from build123d import *

# Parameters (mm, degrees)
EXTRUDE_1_DEPTH     = 12
SKETCH_2_R          = 3
CUT_EXTRUDE_1_DEPTH = 12
FILLET_1_R          = 10
SKETCH_3_R          = 10
CUT_EXTRUDE_2_DEPTH = 12


with BuildPart() as part:
    # 草图1 → 凸台-拉伸1 (new body)
    with BuildSketch(Plane(origin=(0, 0, 0), x_dir=(1, 0, 0), z_dir=(0, 1, 0))):
        with BuildLine():
            Line((-28.145825623, 33.75), (0, 50))
            Line((0, 50), (28.145825623, 33.75))
            ThreePointArc((28.145825623, 33.75), (31.392589354, 41.588381034), (32.5, 50))
            ThreePointArc((32.5, 50), (-8.411618966, 81.392589354), (-28.145825623, 33.75))
        make_face()
        with BuildLine():
            Line((0, 50), (0, 17.5))
            ThreePointArc((0, 17.5), (16.25, 21.854174377), (28.145825623, 33.75))
            Line((28.145825623, 33.75), (0, 50))
        make_face()
        with BuildLine():
            ThreePointArc((-28.145825623, 33.75), (-16.25, 21.854174377), (0, 17.5))
            Line((0, 17.5), (0, 50))
            Line((0, 50), (-28.145825623, 33.75))
        make_face()
        with BuildLine():
            Line((-28.145825623, 0), (0, 0))
            Line((0, 0), (0, 17.5))
            ThreePointArc((0, 17.5), (-16.25, 21.854174377), (-28.145825623, 33.75))
            Line((-28.145825623, 33.75), (-28.145825623, 0))
        make_face()
        with BuildLine():
            Line((0, 17.5), (0, 0))
            Line((0, 0), (28.145825623, 0))
            Line((28.145825623, 0), (28.145825623, 33.75))
            ThreePointArc((28.145825623, 33.75), (16.25, 21.854174377), (0, 17.5))
        make_face()
    extrude(amount=EXTRUDE_1_DEPTH)

    # 草图2 → 切除-拉伸1 (cut)
    with BuildSketch(Plane(origin=(0, 0, 0), x_dir=(-1, 0, 0), z_dir=(0, -1, 0))):
        with Locations(Location((0, 6, 0), (0, 0, 90))):
            Circle(SKETCH_2_R)
        with Locations(Location((20, 6, 0), (0, 0, 90))):
            Circle(SKETCH_2_R)
        with Locations(Location((-20, 6, 0), (0, 0, 90))):
            Circle(SKETCH_2_R)
    extrude(amount=-CUT_EXTRUDE_1_DEPTH, mode=Mode.SUBTRACT)

    # 圆角1
    # the kernel refuses this fillet: 10 mm, written as the material it takes off along each edge
    with BuildSketch(Plane(origin=(-53.145825623, 12, 0), x_dir=(0, 0, -1), z_dir=(1, 0, 0))) as fillet_1_piece_1:
        with BuildLine():
            CenterArc((FILLET_1_R, -FILLET_1_R), FILLET_1_R, 90, 90)
            Line((0, -FILLET_1_R), (0, 0))
            Line((0, 0), (FILLET_1_R, 0))
        make_face()
    extrude(amount=106.291651246, mode=Mode.SUBTRACT)

    # 草图3 → 切除-拉伸2 (cut)
    with BuildSketch(Plane(origin=(0, 12, 0), x_dir=(1, 0, 0), z_dir=(0, 1, 0))):
        with Locations(Location((0, 50, 0), (0, 0, 270))):
            Circle(SKETCH_3_R)
    extrude(amount=-CUT_EXTRUDE_2_DEPTH, mode=Mode.SUBTRACT)


solid = part.part
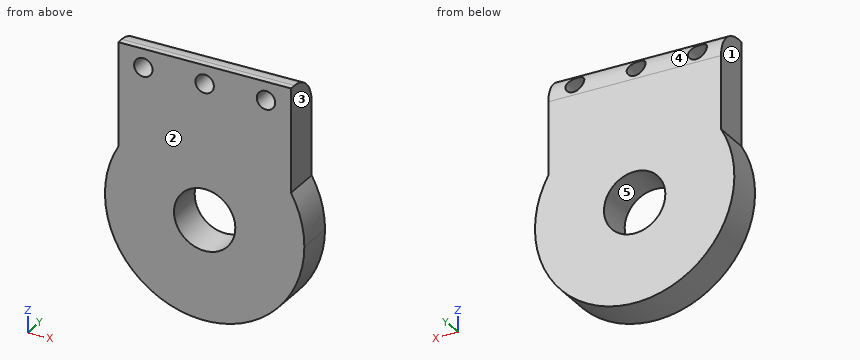
For this review, take the finished solid that the model builds, in its own axes (mm). Face numbers are marked on the shaded views. A direction names the side the tool comes from. Give positions to 0.01 mm unless a question says otherwise; leave off trailing zeros. Order: outer loops, then holes, each group sorted by start corner. A loop starts at its lowest first (then second) coordinate and runs counter-clockwise, first axis right, second up. Notation, with made-up numbers: (40.5, 12) - (50.5, 12) arc R16 cw to (50.5, 30) - close; hole circle Ø1 at (35.5, 74). An arc over 180 degrees is marked (long way). Answer as a JSON object with one key per item and string values. Group by question number.
Item 1: Take a section at C-C on z = -6. Give the boundary of the cut face in (x, y).
Item 2: Take a section at A-A on z = -52. Give the boundary of the cut face in (x, y).
Item 3: Wall thickness on line 1 along X through (y, z) = (3.25, -6); line 2 along X through (y, z) = (3.25, -5); line 3 along Z through (x, y) = (-1, 5.5): over which ranges is each line inside the solid? List them lowest first.
Item 4: Take a section at B-B on x = -20. Give the boundary of the cut face in (y, z).
Item 5: Machinability: for the marked faces 1 and 2, which of the approach directions +Z, -Z, +X, -X, +Y, -Y give a long, thin tool a straight path to every point of the face, cutting with its end or side? Answer none if there is none.
Item 6: Draft analysis for pull direction Z (two halves, no side actions). For the marked faces 3, 4 and 5, state which applies: pulls with the +Z half, pulls with the -Z half, needs draft (parallel to the pull), parting line crosses it, or undercut.
Item 7: Clearance check with flat-ended pins moving along their axes: pin 1 Ø2 at (y, z) = (3.5, -38.5) entering from +X; pin 2 Ø3.5 at (y, z) = (8.5, -15) entering from +X; pin 3 Ø1.5 at (y, z) = (7.5, -10) entering from -X. State where each tip first meets the part, or that it passes through.
Item 8: Take a section at D-D on x = 0. Give the boundary of the cut face in (y, z), and give its area (3 significant figures).
Reported:
{
 "1": {"outline": "(-28.15, 0) - (-23, 0) - (-23, 11.17) - (-28.15, 11.17) - close; (-17, 0) - (-3, 0) - (-3, 11.17) - (-17, 11.17) - close; (3, 0) - (17, 0) - (17, 11.17) - (3, 11.17) - close; (23, 0) - (28.15, 0) - (28.15, 11.17) - (23, 11.17) - close"},
 "2": {"outline": "(-32.44, 0) - (-9.8, 0) - (-9.8, 12) - (-32.44, 12) - close; (9.8, 0) - (32.44, 0) - (32.44, 12) - (9.8, 12) - close"},
 "3": {"line 1": "-28.15 to -23, -17 to -3, 3 to 17, 23 to 28.15", "line 2": "-28.15 to -22.83, -17.17 to -2.83, 2.83 to 17.17, 22.83 to 28.15", "line 3": "-82.48 to -59.95, -40.05 to -8.83, -3.17 to -0.63"},
 "4": {"outline": "(0, -75.62) - (12, -75.62) - (12, -10) arc R10 ccw to (11.95, -9) - (0, -9) - close; (0, -3) - (9.14, -3) arc R10 ccw to (2, 0) - (0, 0) - close"},
 "5": {"face 1": "+Z, -X, +Y, -Y", "face 2": "+Z, -Z, +X, -X, -Y"},
 "6": {"face 3": "needs draft", "face 4": "pulls with the +Z half", "face 5": "undercut"},
 "7": {"pin 1": "x = 30.76", "pin 2": "x = 28.15", "pin 3": "x = -28.15"},
 "8": {"outline": "(0, -82.5) - (12, -82.5) - (12, -60) - (0, -60) - close; (0, -40) - (12, -40) - (12, -10) arc R10 ccw to (11.95, -9) - (0, -9) - close; (0, -3) - (9.14, -3) arc R10 ccw to (2, 0) - (0, 0) - close", "area": "663 mm^2"}
}
